```python
from build123d import *

# Parameters (mm, degrees)
SKETCH1_R           = 2.667
BOSS_EXTRUDE1_DEPTH = 50.8
SKETCH2_R           = 2.667
REVOLVE1_ANGLE      = 52.5
SKETCH3_R           = 2.667
REVOLVE2_ANGLE      = 270
SKETCH4_R           = 2.667
BOSS_EXTRUDE2_DEPTH = 7.62


with BuildPart() as part:
    # Sketch1 → Boss-Extrude1 (new body)
    with BuildSketch(Plane.XY):
        Circle(SKETCH1_R)
    extrude(amount=BOSS_EXTRUDE1_DEPTH)

    # Sketch2 → Revolve1 (revolve)
    with BuildSketch(Plane.XY.offset(50.8)):
        Circle(SKETCH2_R)
    revolve(axis=Axis((-12.192, -2.667, 50.8), (0, -1, 0)), revolution_arc=REVOLVE1_ANGLE)

    # Sketch3 → Revolve2 (revolve)
    with BuildSketch(Plane(origin=(-32.208276887, 0, 24.714280091), x_dir=(0.608761429, 0, 0.79335334), z_dir=(-0.79335334, 0, 0.608761429))):
        with Locations((45.072330344, 0)):
            Circle(SKETCH3_R)
    revolve(axis=Axis((1.105784655, -2.667, 68.130010365), (0, 1, 0)), revolution_arc=REVOLVE2_ANGLE)

    # Sketch4 → Boss-Extrude2 (add)
    with BuildSketch(Plane(origin=(33.314061542, 0, 43.415730274), x_dir=(-0.79335334, 0, 0.608761429), z_dir=(-0.608761429, 0, -0.79335334))):
        with Locations((30.945644518, 0)):
            Circle(SKETCH4_R)
    extrude(amount=BOSS_EXTRUDE2_DEPTH)


solid = part.part
```
Model file for the job. Use its own axes, mm. Coordinates: 2 decimals unless noted, no trailing zeros. Write each loop counter-clockwise with the first axis right and the second up, starting at its lowest first coordinate (ties: lowest second). Pieces come first, ordered by that corner, then holes. Notation, with made-up numbers: (-8.5, 88) - (43.5, 88) arc R9 ccw to (43.5, 103) - close; hole circle Ø7 at (71.5, 82.25). An arc over 180 degrees is marked (long way). One line per item, written item: value. Start each with the question number.
1. Probe line 1 (Z direction, x = 0.25, y = -0.5); line 2 (Z direction, x = 4.25, y = 1.8); line 3 (X direction, y = 1, z = 58). List the from-to ranges inside material, lowest first. Write a range as from..to.
2. Mould opens along X. For faces 1 (the flat face through (0, 0, 0)), 2 (the flat face through (4.15, 0.04, 56.19)), 3 (the cylindrical face through (1.231, -2.366, 25.044)) say: released by +X, released by -X, zero draft, split by the parting line, or undercut.
3. Slice it at A-A (y = 0). Write the cut outline in (x, z) (3 decimals), plus the area to 3 significant figures.
4. Slice it at B-B (z = 49). Write the cut outline in (x, y), plus the area to 3 significant figures.
5. Flat gauge pins, fed straight in: pin 1 (2 mm diameter, centred on y = 0, z = 23, fed in from -X); pin 2 (1 mm diameter, centred on x = -5, y = 0.5, fed in from +Z); pin 3 (2 mm diameter, centred on x = -4.5, y = 1.5, fed in from -Z). Where does each tip first touch, or does it go through?
Answers below:
1. line 1: z = 0..58.84, 75.11..80.37
1. line 2: z = 56.11..59.61, 75.14..79.32
1. line 3: x = -5.66..0.58, 2.38..8.62
2. face 1: zero draft
2. face 2: undercut
2. face 3: split by the parting line
3. outline: (-6.394, 58.357) arc R9.525 cw to (-2.667, 50.8) - (-2.667, 0) - (2.667, 0) - (2.667, 50.8) arc R14.859 ccw to (-3.146, 62.588) arc R6.985 cw (long way) to (6.647, 63.878) - (2.009, 57.832) - (6.24, 54.585) - (10.879, 60.631) arc R12.319 ccw (long way) to start
3. area: 614 mm^2
4. outline: circle Ø5.33 at (0, 0)
4. area: 22.3 mm^2
5. pin 1: stops at x = -2.67
5. pin 2: stops at z = 79.06
5. pin 3: stops at z = 55.4
